Autodesk Inventor part; units mm, degrees
ref_plane "YZ Plane" through (0, 0, 0) normal (1, 0, 0) x (0, 1, 0)
ref_plane "XZ Plane" through (0, 0, 0) normal (0, 1, 0) x (-1, 0, 0)
ref_plane "XY Plane" through (0, 0, 0) normal (0, 0, 1) x (1, 0, 0)
ref_plane "Work Plane1" through (0, 0, 0) normal (0, 0, 1) x (1, 0, 0)
sketch "Sketch1" plane through (0, 0, 0) normal (0, 0, 1) x (1, 0, 0)
  circle A0 centre (6.5, 20.75) radius 1
  circle A1 centre (6.5, 4.75) radius 1
  circle A2 centre (22.5, 20.75) radius 1
  circle A3 centre (22.5, 4.75) radius 1
  line L0 (-13, -14.75) -> (42, -14.75)
  line L1 (42, -14.75) -> (42, 40.25)
  line L2 (42, 40.25) -> (-13, 40.25)
  line L3 (-13, 40.25) -> (-13, -14.75)
  line L4 (-13, -14.75) -> (42, 40.25) construction
  line L5 (42, -14.75) -> (-13, 40.25) construction
  circle A4 centre (22.5, 12.75) radius 1
  circle A5 centre (14.5, 20.75) radius 1
  circle A6 centre (14.5, 4.75) radius 1
  circle A7 centre (6.5, 12.75) radius 1
  line L6 (19.5, 15.75) -> (19.5, 9.75)
  line L7 (17.1458, 15.75) -> (19.5, 15.75)
  arc A8 (17.1458, 15.75) -> (11.8542, 15.75) centre (14.5, 12.75) ccw
  line L8 (9.5, 15.75) -> (11.8542, 15.75)
  line L9 (9.5, 9.75) -> (9.5, 15.75)
  line L10 (11.8542, 9.75) -> (9.5, 9.75)
  arc A9 (11.8542, 9.75) -> (17.1458, 9.75) centre (14.5, 12.75) ccw
  line L11 (19.5, 9.75) -> (17.1458, 9.75)
  point P0 (0, 0)
  dimension "d0" = 55
  dimension "d1" = 55
  dimension "d95" = 2
  dimension "d96" = 2
  dimension "d97" = 2
  dimension "d98" = 2
extrude "Extrusion3" add sketch "Sketch1" along normal blind 3
sketch "Sketch4" plane through (0, 0, 3) normal (0, 0, 1) x (1, 0, 0)
  line L0 (14.5, 40.25) -> (14.5, 12.75) construction
  line L1 (-13, -14.75) -> (42, -14.75) construction
  line L2 (-13, 12.75) -> (14.5, 12.75) construction
  line L3 (5, 38.25) -> (-7, 38.25)
  line L4 (-7, 38.25) -> (-7, 33.25)
  line L5 (-7, 33.25) -> (13, 33.25)
  line L6 (13, 40.25) -> (13, 33.25)
  line L7 (-7, -12.75) -> (5, -12.75)
  line L8 (5, -12.75) -> (5, -7.75)
  line L9 (5, -7.75) -> (-13, -7.75)
  line L10 (-13, -14.75) -> (-13, -7.75)
  line L11 (-13, -14.75) -> (5.3284, -14.75)
  line L12 (14.5, 12.75) -> (20.6229, 27.5321)
  line L13 (14.5, 12.75) -> (30.5, 12.75) construction
  circle A0 centre (20.6229, 27.5321) radius 3.895
  circle A1 centre (8.3771, 27.5321) radius 3.895
  circle A2 centre (-0.2821, 18.8729) radius 3.895
  circle A3 centre (-0.2821, 6.6271) radius 3.895
  circle A4 centre (8.3771, -2.0321) radius 3.895
  circle A5 centre (20.6229, -2.0321) radius 3.895
  circle A6 centre (29.2821, 6.6271) radius 3.895
  circle A7 centre (29.2821, 18.8729) radius 3.895
  line L14 (-7, -12.75) -> (-7, -9.75)
  line L15 (-7, -9.75) -> (-13, -9.75)
  line L16 (-13, 40.25) -> (-13, -14.75)
  line L17 (-13, -7.75) -> (-13, -9.75)
  line L18 (-13, 40.25) -> (-13, -14.75)
  line L19 (5, 38.25) -> (5, 35.25)
  line L20 (5, 35.25) -> (11, 35.25)
  line L21 (11, 35.25) -> (11, 40.25)
  line L22 (42, 40.25) -> (-13, 40.25)
  line L23 (42, 40.25) -> (-13, 40.25)
  line L24 (11, 40.25) -> (13, 40.25)
  line L25 (24, 38.25) -> (36, 38.25)
  line L26 (36, 38.25) -> (36, 33.25)
  line L27 (36, 33.25) -> (16, 33.25)
  line L28 (16, 40.25) -> (16, 33.25)
  line L29 (24, 38.25) -> (24, 35.25)
  line L30 (24, 35.25) -> (18, 35.25)
  line L31 (18, 35.25) -> (18, 40.25)
  line L32 (18, 40.25) -> (16, 40.25)
  point P0 (0, 0)
  dimension "d99" = 16
  dimension "d100" = 67.5
  dimension "d101" = 7.79
  dimension "d104" = 360
  dimension "d106" = 2
  dimension "d107" = 5
  dimension "d108" = 2
  dimension "d109" = 12
  dimension "d110" = 18
  dimension "d111" = 6
  dimension "d112" = 20
  dimension "d113" = 12
  dimension "d114" = 6
  dimension "d115" = 5
  dimension "d117" = 2
  dimension "d118" = 2
extrude "Extrusion2" cut sketch "Sketch4" against normal through all
fillet "Fillet3" radius 2 14 edges at (-7, 38.25, 1.5) (5, 38.25, 1.5) (13, 33.25, 1.5) (5, -12.75, 1.5) (-7, -12.75, 1.5) (-7, -9.75, 1.5) (-13, -9.75, 1.5) (5, 35.25, 1.5) (11, 35.25, 1.5) (18, 35.25, 1.5) (24, 35.25, 1.5) (24, 38.25, 1.5) (36, 38.25, 1.5) (16, 33.25, 1.5)
sketch "Sketch6" plane through (0, 0, 3) normal (0, 0, 1) x (1, 0, 0)
  line L0 (38.85, 20.3) -> (42, 20.3)
  line L1 (42, 20.3) -> (42, 5.2)
  line L2 (42, 5.2) -> (38.85, 5.2)
  line L3 (38.85, 5.2) -> (38.85, 20.3)
  line L4 (42, -14.75) -> (42, 40.25)
  line L5 (42, 40.25) -> (-13, 40.25) construction
  line L6 (14.5, 40.25) -> (14.5, -14.75) construction
  line L7 (-13, -14.75) -> (42, -14.75) construction
  line L8 (-9.85, 20.3) -> (-13, 20.3)
  line L9 (-13, 5.2) -> (-9.85, 5.2)
  line L10 (-9.85, 5.2) -> (-9.85, 20.3)
  line L11 (-13, 12.75) -> (42, 12.75) construction
  line L12 (-13, 20.3) -> (-13, 5.2)
  line L13 (-13, 40.25) -> (-13, -14.75)
  point P0 (0, 0)
  point P1 (42, 12.75)
  point P2 (18.0284, 40.25)
  point P3 (13, 40.25)
  point P4 (5.3284, -14.75)
  point P5 (-13, 12.75)
  point P6 (-13, -7.75)
  dimension "d91" = 3.15
  dimension "d92" = 15.1
extrude "Extrusion4" cut sketch "Sketch6" against normal through all
equation "\"d38\" = d24"
properties part number "BottomRotated"
Work out the finished part from the listing and answer in its coordinate system (mm). A direction names the side the tool comes from. Round coordinates to 2 decimals unless told otherwise and drop trailing zeros. Loops run counter-clockwise (first coordinate to the right, second up) from the corner with the lowest first, then second, coordinate; pieces in that order, holes last. Notation, with made-up numbers: M 9,-12 L 68,-12 A16 ccw 68,-3 Z; hole C -12,81 d7. An arc over 180 degrees is marked long. Use CSV: the item, a comma, the result in double quotes.
Q1. The mould has two halves that part along Y. Classify faces 1 (the flat face through (14, -14.75, 1)), 2 (the flat face through (9.5, 13, 1)), 3 (the flat face through (42, -5, 1)): pulls with the +Y half, pulls with the -Y half, needs draft (parallel to the pull), parting line crosses it, or undercut.
Determined:
face 1,"pulls with the -Y half"
face 2,"undercut"
face 3,"needs draft"
Q2. Section C-C, the plane x = 0.5 is taken. Determine the outline of the cut face in (y, z), then the cut area to 3 significant figures.
Determined:
outline,"M -14.75,0 L -12.75,0 L -12.75,3 L -14.75,3 Z; M -7.75,0 L 2.81,0 L 2.81,3 L -7.75,3 Z; M 10.44,0 L 15.06,0 L 15.06,3 L 10.44,3 Z; M 22.69,0 L 33.25,0 L 33.25,3 L 22.69,3 Z; M 38.25,0 L 40.25,0 L 40.25,3 L 38.25,3 Z"
area,"89.2 mm2"
Q3. A tool of negligible diameter and unlimited length cuts with its end or side. For faces 4 (the flat face through (11, 39, 2)), 5 (the flat face through (-11, 5.2, 2)), 6 (the flat face through (30, 38.25, 2)), 7 (the flat face through (40, 20.3, 2)), from which of +Z, -Z, +X, -X, +Y, -Y can it reach the whole face along a straight path? Write none if from no direction.
Determined:
face 4,"+Z, -Z, +Y"
face 5,"+Z, -Z, -X"
face 6,"+Z, -Z"
face 7,"+Z, -Z, +X"
Q4. Consider L1, parallel to Y at x = -10, z = 1.45; L2, parallel to X at y = 7, z = 2 (3 decimals); L3, parallel to Y at x = 21, z = 1.35. Determine where each line is inside the solid, lowest interval first.
Determined:
L1,"-14.75 to -9.75, -7.75 to 5.2, 20.3 to 40.25"
L2,"-9.85 to -4.159, 3.595 to 25.405, 33.159 to 38.85"
L3,"-14.75 to -5.91, 1.84 to 23.66, 31.41 to 33.25, 35.25 to 40.25"
Q5. Section A-A, the plane x = 14.5 is taken. Determine the outline of the cut face in (y, z), then the cut area to 3 significant figures.
Determined:
outline,"M -14.75,0 L 3.75,0 L 3.75,3 L -14.75,3 Z; M 5.75,0 L 8.75,0 L 8.75,3 L 5.75,3 Z; M 16.75,0 L 19.75,0 L 19.75,3 L 16.75,3 Z; M 21.75,0 L 40.25,0 L 40.25,3 L 21.75,3 Z"
area,"129 mm2"
Q6. Section B-B, the plane y = 12.75 is taken. Determine the outline of the cut face in (x, z).
Determined:
outline,"M -9.85,0 L 5.5,0 L 5.5,3 L -9.85,3 Z; M 7.5,0 L 9.5,0 L 9.5,3 L 7.5,3 Z; M 19.5,0 L 21.5,0 L 21.5,3 L 19.5,3 Z; M 23.5,0 L 38.85,0 L 38.85,3 L 23.5,3 Z"
Q7. Section D-D, the plane y = 26.5 is taken. Determine the outline of the cut face in (x, z).
Determined:
outline,"M -13,0 L 4.62,0 L 4.62,3 L -13,3 Z; M 12.13,0 L 16.87,0 L 16.87,3 L 12.13,3 Z; M 24.38,0 L 42,0 L 42,3 L 24.38,3 Z"
